Work out the finished part from the listing and answer in its coordinate system (mm). A direction names the side the tool comes from. Round coordinates to 2 decimals unless told otherwise and drop trailing zeros. Loops run counter-clockwise (first coordinate to the right, second up) from the corner with the lowest first, then second, coordinate; pieces in that order, holes last. Notation, with made-up numbers: (-1, 65.5) -> (33, 65.5) arc R6 cw to (33, 74.5) -> close; hole circle Ø6 at (64, 44.5). An arc over 180 degrees is marked (long way). Write item = value, one per line. Start each with the question number.
```python
from build123d import *

# Parameters (mm, degrees)
F0_W         = 127
F0_H         = 50.8
F1_DEPTH     = 38.1
F2_T1_DEPTH  = 57.15
F2_T3_DEPTH  = 114.3
F2_T5_DEPTH  = 25.4
F2_T7_DEPTH  = 146.05
F2_S11_W     = 12.7
F2_S11_H     = 12.7
F2_T12_DEPTH = 12.7
F2_S17_W     = 12.7
F2_S17_H     = 12.7
F2_T18_DEPTH = 12.7


# Not quite as in the source:
# - a fillet or chamfer that OpenCascade refuses, or shapes differently, is made with other operations: its cross-section is extruded or revolved along the edge and cut away or added


with BuildPart() as f1:
    # F0 (on Top) → F1 (new body)
    with BuildSketch(Plane.XY):
        with Locations((4.3936092407, 0)):
            Rectangle(F0_W, F0_H)
        Polygon((-28.6239193533, -16.7126883595), (-52.4921119213, 0), (-28.6239193533, 8.6873116405), align=None, mode=Mode.SUBTRACT)
    extrude(amount=F1_DEPTH)

    # F2: fillet of radius 12.7 on 6 edges, made by hand

    # F2_s2 → F2_t1 (cut)
    with BuildSketch(Plane.XY.offset(-31.75)):
        with BuildLine():
            ThreePointArc((-46.4063907593, 25.4), (-55.3866468804, 21.6802561211), (-59.1063907593, 12.7))
            Line((-59.1063907593, 12.7), (-59.1063907593, 25.4))
            Line((-59.1063907593, 25.4), (-46.4063907593, 25.4))
        make_face()
        with BuildLine():
            ThreePointArc((-59.1063907593, -12.7), (-55.3866468804, -21.6802561211), (-46.4063907593, -25.4))
            Line((-46.4063907593, -25.4), (-59.1063907593, -25.4))
            Line((-59.1063907593, -25.4), (-59.1063907593, -12.7))
        make_face()
    extrude(amount=F2_T1_DEPTH, mode=Mode.SUBTRACT)

    # F2_s4 → F2_t3 (cut)
    with BuildSketch(Plane.XZ.offset(-57.15)):
        with BuildLine():
            ThreePointArc((-59.1063907593, 12.7), (-55.3866468804, 3.7197438789), (-46.4063907593, 0))
            Line((-46.4063907593, 0), (-59.1063907593, 0))
            Line((-59.1063907593, 0), (-59.1063907593, 12.7))
        make_face()
    extrude(amount=F2_T3_DEPTH, mode=Mode.SUBTRACT)

    # F2_s6 → F2_t5 (cut)
    with BuildSketch(Plane.XZ.offset(-12.7)):
        with BuildLine():
            ThreePointArc((-59.1063907593, 25.4), (-55.3866468804, 34.3802561211), (-46.4063907593, 38.1))
            Line((-46.4063907593, 38.1), (-59.1063907593, 38.1))
            Line((-59.1063907593, 38.1), (-59.1063907593, 25.4))
        make_face()
    extrude(amount=F2_T5_DEPTH, mode=Mode.SUBTRACT)

    # F2_s8 → F2_t7 (cut)
    with BuildSketch(Plane.YZ.offset(-46.4063907593)):
        with BuildLine():
            ThreePointArc((-25.4, 25.4), (-21.6802561211, 34.3802561211), (-12.7, 38.1))
            Line((-12.7, 38.1), (-25.4, 38.1))
            Line((-25.4, 38.1), (-25.4, 25.4))
        make_face()
        with BuildLine():
            ThreePointArc((25.4, 25.4), (21.6802561211, 34.3802561211), (12.7, 38.1))
            Line((12.7, 38.1), (25.4, 38.1))
            Line((25.4, 38.1), (25.4, 25.4))
        make_face()
    extrude(amount=F2_T7_DEPTH, mode=Mode.SUBTRACT)


with BuildPart() as f2_tool10:
    # F2_s11 → F2_t12 (new body)
    with BuildSketch(Plane.XZ.offset(-12.7)):
        with Locations((-52.7563907593, 31.75)):
            Rectangle(F2_S11_W, F2_S11_H)
    extrude(amount=-F2_T12_DEPTH)

    # F2_s13 → F2_t14 (revolve, cut)
    with BuildSketch(Plane(origin=(-46.4063907593, 12.7, 25.4), x_dir=(0.7071067812, 0, -0.7071067812), z_dir=(0.7071067812, 0, 0.7071067812))):
        with BuildLine():
            ThreePointArc((0, -12.7), (12.7, 0), (0, 12.7))
            Line((0, 12.7), (0, -12.7))
        make_face()
    revolve(axis=Axis((-46.4063907593, 12.7, 25.4), (0, 1, 0)), mode=Mode.SUBTRACT)


with BuildPart() as f1_1:
    add(f1.part)

    # F2_t9: cut F2_tool10
    add(f2_tool10.part, mode=Mode.SUBTRACT)


with BuildPart() as f2_tool16:
    # F2_s17 → F2_t18 (new body)
    with BuildSketch(Plane.XY.offset(25.4)):
        with Locations((-52.7563907593, -19.05)):
            Rectangle(F2_S17_W, F2_S17_H)
    extrude(amount=F2_T18_DEPTH)

    # F2_s19 → F2_t20 (revolve, cut)
    with BuildSketch(Plane(origin=(-46.4063907593, -12.7, 25.4), x_dir=(0.7071067812, 0.7071067812, 0), z_dir=(0.7071067812, -0.7071067812, 0))):
        with BuildLine():
            ThreePointArc((0, -12.7), (12.7, 0), (0, 12.7))
            Line((0, 12.7), (0, -12.7))
        make_face()
    revolve(axis=Axis((-46.4063907593, -12.7, 25.4), (0, 0, 1)), mode=Mode.SUBTRACT)


with BuildPart() as f1_2:
    add(f1_1.part)

    # F2_t15: cut F2_tool16
    add(f2_tool16.part, mode=Mode.SUBTRACT)


solid = f1_2.part
```
Item 1: A tool of negligible diameter and unlimited length cuts with its end or side. For faces 5 (the flat face through (10, -25.4, 13)), 6 (the flat face through (-40.73, 4.28, 18.78)), from which of +Z, -Z, +X, -X, +Y, -Y can it reach the whole face along a straight path? Write none if from no direction.
Item 2: Section A-A (y = -15.5) is taken. Determine the outline of the cut face in (x, z), then the cut area to 3 significant figures.
Item 3: Section B-B (z = 34) is taken. Determine the outline of the cut face in (x, y).
Item 4: The mould has two halves that part along X. Classify faces 1 (the flat face through (-43, -10, 38.1)), 2 (the flat face through (67.894, 0, 19)), 3 (the flat face through (-40.391, -8.473, 18.783)), 4 (the cylindrical face through (-55.485, 0.356, 3.819)): pulls with the +X half, pulls with the -X half, needs draft (parallel to the pull), parting line crosses it, or undercut.
Item 5: Section C-C (x = 58) is taken. Determine the outline of the cut face in (y, z).
Item 6: Section D-D (y = 21) is taken. Determine the outline of the cut face in (x, z).
Item 7: Find the intervals of material crossed by line 1 along X through (y, z) = (-11, 11); line 2 along Y through (x, z) = (43.5, 25.5); line 3 along X through (y, z) = (-2, 9.5), in increasing order. Write a range as [from, to].
Item 8: Flat-ended cylindrical pins translate along their axes: pin 1 (1 mm diameter, centred on y = 11, z = 10, fed in from -X); pin 2 (1.5 mm diameter, centred on x = 20.5, z = 27, fed in from -Y); pin 3 (1 mm diameter, centred on x = -10.5, z = 28, fed in from +Y). Find the tip coordinate at first contact, or state that the pin passes through.
Worked answers:
q1.face_5 = +Z, -Z, +X, -X, -Y
q1.face_6 = +Z, -Z
q2.outline = (-58.79, 9.9) arc R12.7 ccw to (-46.41, 0) -> (-30.36, 0) -> (-30.36, 37.79) -> (-46.41, 37.79) arc R12.39 ccw to (-58.79, 25.4) -> close; (-28.62, 0) -> (67.89, 0) -> (67.89, 37.79) -> (-28.62, 37.79) -> close
q2.area = 4,660 mm2
q3.outline = (-55.75, -12.7) arc R9.35 ccw to (-46.41, -22.05) -> (67.89, -22.05) -> (67.89, 22.05) -> (-46.41, 22.05) arc R9.35 ccw to (-55.75, 12.7) -> close; hole (-52.49, 0) -> (-28.62, -16.71) -> (-28.62, 8.69) -> close
q4.face_1 = needs draft
q4.face_2 = pulls with the +X half
q4.face_3 = undercut
q4.face_4 = pulls with the -X half
q5.outline = (-25.4, 0) -> (25.4, 0) -> (25.4, 25.4) arc R12.7 ccw to (12.7, 38.1) -> (-12.7, 38.1) arc R12.7 ccw to (-25.4, 25.4) -> close
q6.outline = (-56.02, 4.4) arc R12.7 ccw to (-46.41, 0) -> (67.89, 0) -> (67.89, 35.01) -> (-46.41, 35.01) arc R9.61 ccw to (-56.02, 25.4) -> close
q7.line_1 = [-58.99, -36.78], [-28.62, 67.89]
q7.line_2 = [-25.4, 25.4]
q7.line_3 = [-58.7, -49.64], [-28.62, 67.89]
q8.pin_1 = -58.91
q8.pin_2 = -25.37
q8.pin_3 = 25.23
